from build123d import *

# Parameters (mm, degrees)
SKETCH2_W           = 19.05
SKETCH2_H           = 19.05
SKETCH2_W_2         = 15.875
SKETCH2_H_2         = 15.875
BOSS_EXTRUDE1_DEPTH = 400
FILLET1_R           = 1


with BuildPart() as part:
    # Sketch2 → Boss-Extrude1 (new body)
    with BuildSketch(Plane(origin=(0, 0, 0), x_dir=(0, 0, -1), z_dir=(1, 0, 0))):
        Rectangle(SKETCH2_W, SKETCH2_H)
        Rectangle(SKETCH2_W_2, SKETCH2_H_2, mode=Mode.SUBTRACT)
    extrude(amount=BOSS_EXTRUDE1_DEPTH)

    # Fillet1
    fillet1_edges = [part.edges().sort_by_distance(p)[0] for p in [
        (200, -9.525, -9.525),
        (200, -9.525, 9.525),
        (200, 9.525, 9.525),
        (200, 9.525, -9.525),
    ]]
    fillet(fillet1_edges, radius=FILLET1_R)


solid = part.part
Could you check a few things on this model? Use its own coordinates, in mm. A direction names the side the tool comes from. Coordinates: 2 decimals unless noted, no trailing zeros. Loops run counter-clockwise (first coordinate to the right, second up) from the corner with the lowest first, then second, coordinate; pieces in that order, holes last.
1. Imagine slicing it at A-A (y = -3.5). Please give me the cut outline in (x, z) (1 decimal).
2. I need wall thicknesses on L1, parallel to Y at x = 46, z = -5.5 (1 decimal). Which ranges of the line are inside material? Lowest first, please.
3. We'd pull the mould along Z, two halves only. Please class faces 1 (the face through (197, 0, -9.525)), 2 (the face through (197, 0, 9.525)), 3 (the face through (197, 0, -7.938)), 4 (the face through (400, 0, 9)): released by +Z, released by -Z, zero draft, split by the parting line, or undercut.
4. For P1, Ø1, axis at y = 6, z = 6.5, coming from the +X side, with a flat end and sliding along its axis, tell me the tip position at first contact or that it passes through.
5. Imagine slicing it at C-C (x = 74). Please give me the cut outline in (y, z) (1 decimal), and give its area (3 significant figures).
6. For faces 5 (the face through (197, 7.938, 0)), 6 (the face through (197, -9.525, 0)), which set-ups out of +Z, -Z, +X, -X, +Y, -Y let a thin tool reach every point of the face, with its end or its side?
Computed values:
1. outline: (0, -9.5) - (400, -9.5) - (400, -7.9) - (0, -7.9) - close; (0, 7.9) - (400, 7.9) - (400, 9.5) - (0, 9.5) - close
2. L1: y = -9.5 to -7.9, 7.9 to 9.5
3. face 1: released by -Z
3. face 2: released by +Z
3. face 3: undercut
3. face 4: zero draft
4. P1: passes through
5. outline: (-9.5, -8.5) arc R1 ccw to (-8.5, -9.5) - (8.5, -9.5) arc R1 ccw to (9.5, -8.5) - (9.5, 8.5) arc R1 ccw to (8.5, 9.5) - (-8.5, 9.5) arc R1 ccw to (-9.5, 8.5) - close; hole (-7.9, -7.9) - (7.9, -7.9) - (7.9, 7.9) - (-7.9, 7.9) - close
5. area: 110 mm2
6. face 5: +X, -X
6. face 6: +Z, -Z, +X, -X, -Y
